```python
from build123d import *

# Parameters (mm, degrees)
SKETCH1_R           = 87.5
SKETCH1_R_2         = 2
SKETCH1_W           = 20
SKETCH1_H           = 41
SKETCH1_W_2         = 18
SKETCH1_H_2         = 8
SKETCH1_W_3         = 8
SKETCH1_H_3         = 18
SKETCH1_W_4         = 9
SKETCH1_H_4         = 4
SKETCH1_W_5         = 4
SKETCH1_H_5         = 9
BOSS_EXTRUDE2_DEPTH = 10


with BuildPart() as part:
    # Sketch1 → Boss-Extrude2 (new body)
    with BuildSketch(Plane.XY):
        with Locations((-18.556626979, 51.967802173)):
            Circle(SKETCH1_R)
        with Locations((41.943373021, 85.967802173)):
            Circle(SKETCH1_R_2, mode=Mode.SUBTRACT)
        with Locations((51.943373021, 85.967802173)):
            Circle(SKETCH1_R_2, mode=Mode.SUBTRACT)
        with Locations((-12.556626979, 86.967802173)):
            Circle(SKETCH1_R_2, mode=Mode.SUBTRACT)
        with Locations(Location((-24.556626979, 86.967802173, 0), (0, 0, 180))):
            Circle(SKETCH1_R_2, mode=Mode.SUBTRACT)
        with Locations(Location((-12.556626979, 37.967802173, 0), (0, 0, 180))):
            Circle(SKETCH1_R_2, mode=Mode.SUBTRACT)
        with Locations((-24.556626979, 37.967802173)):
            Circle(SKETCH1_R_2, mode=Mode.SUBTRACT)
        with Locations(Location((51.943373021, 17.967802173, 0), (0, 0, 180))):
            Circle(SKETCH1_R_2, mode=Mode.SUBTRACT)
        with Locations(Location((41.943373021, 17.967802173, 0), (0, 0, 180))):
            Circle(SKETCH1_R_2, mode=Mode.SUBTRACT)
        with Locations(Location((-89.056626979, 85.967802173, 0), (0, 0, 180))):
            Circle(SKETCH1_R_2, mode=Mode.SUBTRACT)
        with Locations(Location((-79.056626979, 85.967802173, 0), (0, 0, 180))):
            Circle(SKETCH1_R_2, mode=Mode.SUBTRACT)
        with Locations((-79.056626979, 17.967802173)):
            Circle(SKETCH1_R_2, mode=Mode.SUBTRACT)
        with Locations((-89.056626979, 17.967802173)):
            Circle(SKETCH1_R_2, mode=Mode.SUBTRACT)
        with Locations((-18.556626979, 62.467802173)):
            Rectangle(SKETCH1_W, SKETCH1_H, mode=Mode.SUBTRACT)
        with Locations((-18.556626979, -15.532197827)):
            Rectangle(SKETCH1_W_2, SKETCH1_H_2, mode=Mode.SUBTRACT)
        with Locations((-18.556626979, 119.467802173)):
            Rectangle(SKETCH1_W_2, SKETCH1_H_2, mode=Mode.SUBTRACT)
        with Locations((-86.056626979, 51.967802173)):
            Rectangle(SKETCH1_W_3, SKETCH1_H_3, mode=Mode.SUBTRACT)
        with Locations((48.943373021, 51.967802173)):
            Rectangle(SKETCH1_W_3, SKETCH1_H_3, mode=Mode.SUBTRACT)
        with Locations((-18.556626979, 131.467802173)):
            Rectangle(SKETCH1_W_4, SKETCH1_H_4, mode=Mode.SUBTRACT)
        with Locations((-18.556626979, 107.467802173)):
            Rectangle(SKETCH1_W_4, SKETCH1_H_4, mode=Mode.SUBTRACT)
        with Locations((-18.556626979, -27.532197827)):
            Rectangle(SKETCH1_W_4, SKETCH1_H_4, mode=Mode.SUBTRACT)
        with Locations((-18.556626979, -3.532197827)):
            Rectangle(SKETCH1_W_4, SKETCH1_H_4, mode=Mode.SUBTRACT)
        with Locations((60.943373021, 51.967802173)):
            Rectangle(SKETCH1_W_5, SKETCH1_H_5, mode=Mode.SUBTRACT)
        with Locations((36.943373021, 51.967802173)):
            Rectangle(SKETCH1_W_5, SKETCH1_H_5, mode=Mode.SUBTRACT)
        with Locations((-74.056626979, 51.967802173)):
            Rectangle(SKETCH1_W_5, SKETCH1_H_5, mode=Mode.SUBTRACT)
        with Locations((-98.056626979, 51.967802173)):
            Rectangle(SKETCH1_W_5, SKETCH1_H_5, mode=Mode.SUBTRACT)
    extrude(amount=BOSS_EXTRUDE2_DEPTH)


solid = part.part
```
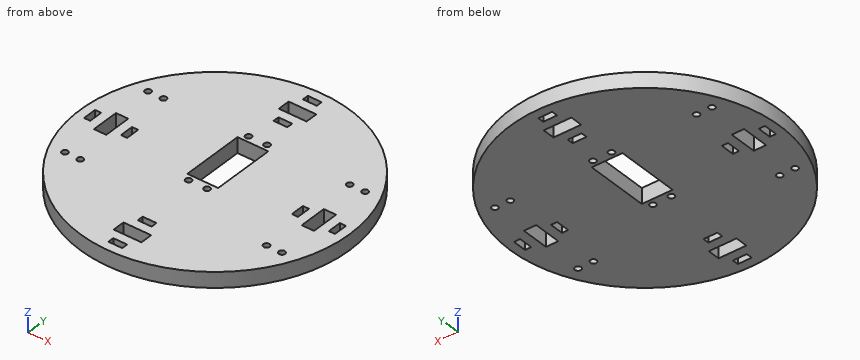
Can you work these out from the model? Positions are in its coordinate system, mm. Coordinates: 2 decimals unless noted, no trailing zeros. Loops run counter-clockwise (first coordinate to the right, second up) from the corner with the lowest first, then second, coordinate; pieces in that order, holes last. Notation, with made-up numbers: (-18.5, 60) - (-6.5, 60) arc R26 ccw to (-6.5, 91) - close; hole circle Ø10 at (-1, 60). An arc over 180 degrees is marked (long way). Answer as CSV lines item,"result". Start each with the question number.
1) I need wall thicknesses on line 1 (X direction, y = 39.5, z = 7); line 2 (Y direction, x = -84.5, z = 4.5) (3 decimals); line 3 (Y direction, x = 43.5, z = 8). Which ranges of each line are inside material? Lowest first, please. Write a range as from..to.
2) Suppose I cut it at A-A (x = -35.5). Please give me the cut outline in (y, z).
3) For pin 1 (1.5 mm diameter, centred on y = -12.5, z = 6, fed in from -X); pin 2 (6 mm diameter, centred on x = -70, z = 3.5, fed in from -Y); pin 3 (2.5 mm diameter, centred on x = -86.5, z = 5, fed in from -Y), each with a flat end and sliding along its axis, tell me the tip position at first contact or that it passes through.
4) Suppose I cut it at B-B (z = 4). Count the separate pieces of the cut face and the enclosed holes in it, plus the area to 3 significant figures.
5) Suppose I cut it at C-C (x = 12). Please give me the cut outline in (y, z), plus the area to 3 significant figures.
Check result:
1,line 1,"x = -105.16..-25.84, -23.27..-13.84, -11.27..68.05"
1,line 2,"y = -5.545..42.968, 60.968..109.481"
1,line 3,"y = -9.72..16.71, 19.22..84.71, 87.22..113.65"
2,outline,"(-33.88, 0) - (137.81, 0) - (137.81, 10) - (-33.88, 10) - close"
3,pin 1,"stops at x = -78.53"
3,pin 2,"stops at y = -20.9"
3,pin 3,"stops at y = -4.67"
4,separate pieces,"1"
4,enclosed holes,"25"
4,area,"22,200 mm²"
5,outline,"(-30.02, 0) - (133.96, 0) - (133.96, 10) - (-30.02, 10) - close"
5,area,"1,640 mm²"
